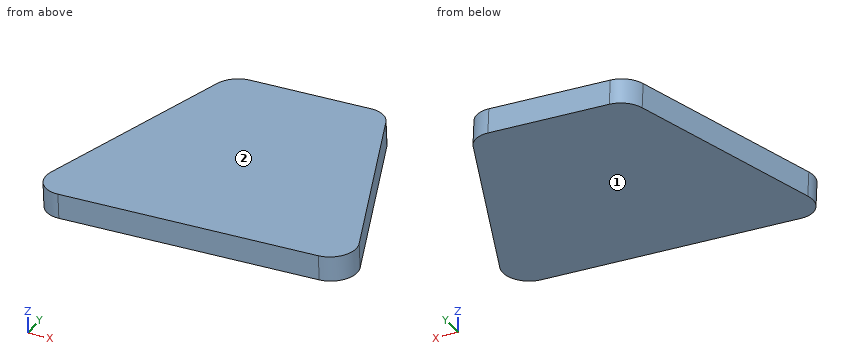
from build123d import *

# Parameters (mm, degrees)
BOSS_EXTRUDE1_DEPTH = 2.54
FILLET1_R           = 2.54


with BuildPart() as part:
    # Sketch1 → Boss-Extrude1 (new body)
    with BuildSketch(Plane(origin=(-8.073375318, 5.240605229, 134.378875143), x_dir=(0.998202842, 0.00233525, 0.059880156), z_dir=(-0.059925675, 0.038899072, 0.997444623))):
        Polygon((16.485952237, 500.26984873), (26.498547321, 474.86984873), (-7.418569241, 474.86984873), (0.410574683, 500.26984873), align=None)
    extrude(amount=BOSS_EXTRUDE1_DEPTH)

    # Fillet1
    fillet1_edges = [part.edges().sort_by_distance(p)[0] for p in [
        (8.306843448, 505.218357591, 117.137742749),
        (18.301444315, 479.861032939, 118.727113786),
        (-15.554717825, 479.781827994, 116.696151541),
        (-7.73964411, 505.180817566, 116.175146627),
    ]]
    fillet(fillet1_edges, radius=FILLET1_R)


solid = part.part
The model under review builds one solid part; all positions refer to its coordinate system, in mm. Face numbers are marked on the shaded views. Coordinates: 2 decimals unless noted, no trailing zeros. Write each loop counter-clockwise with the first axis right and the second up, starting at its lowest first coordinate (ties: lowest second). Pieces come first, ordered by that corner, then holes. Notation, with made-up numbers: (51.25, -12) - (103.25, -12) arc R16 cw to (103.25, -5) - close; hole circle Ø10 at (56.5, -17.5). An arc over 180 degrees is marked (long way). Answer as a JSON object with one key per item and string values. Group by question number.
1. Add section B-B (x = 3). Give the boundary of the cut face in (y, z), plus the area to 3 significant figures.
2. Clearance check with flat-ended pins moving along their axes: pin 1 Ø1.5 at (x, y) = (0.5, 483.5) entering from -Z; pin 2 Ø5 at (x, y) = (-5.5, 483) entering from +Z. State where each tip first meets the part, or that it passes through.
3. Mouldability with a two-part tool opening along Z and no side actions: class the marked faces 1 and 2 as pulls with the +Z half, pulls with the -Z half, needs draft (parallel to the pull), parting line crosses it, or undercut.
4. Add section A-A (y = 488.75). Give the boundary of the cut face in (x, z), plus the area to 3 significant figures.
5. To check wall thickness, follow probe 1 along X at (y, z) = (493, 116.85); probe 2 along Z at (x, y) = (5, 502.75); probe 3 along X at (y, z) = (497.25, 116.9). State the ranges of each line that lie inside material, in increasing order.
Findings:
{
 "1": {"outline": "(479.78, 116.54) - (505.16, 115.55) - (505.26, 118.09) - (479.87, 119.08) - close", "area": "64.6 mm²"},
 "2": {"pin 1": "z = 116.19", "pin 2": "z = 118.63"},
 "3": {"face 1": "pulls with the -Z half", "face 2": "pulls with the +Z half"},
 "4": {"outline": "(-12.89, 117.78) - (-12.7, 115.24) - (14.85, 116.9) - (14.74, 119.44) - close", "area": "70.3 mm²"},
 "5": {"probe 1": "-11.52 to 13.17", "probe 2": "115.76 to 118.31", "probe 3": "-10.22 to 11.48"}
}
